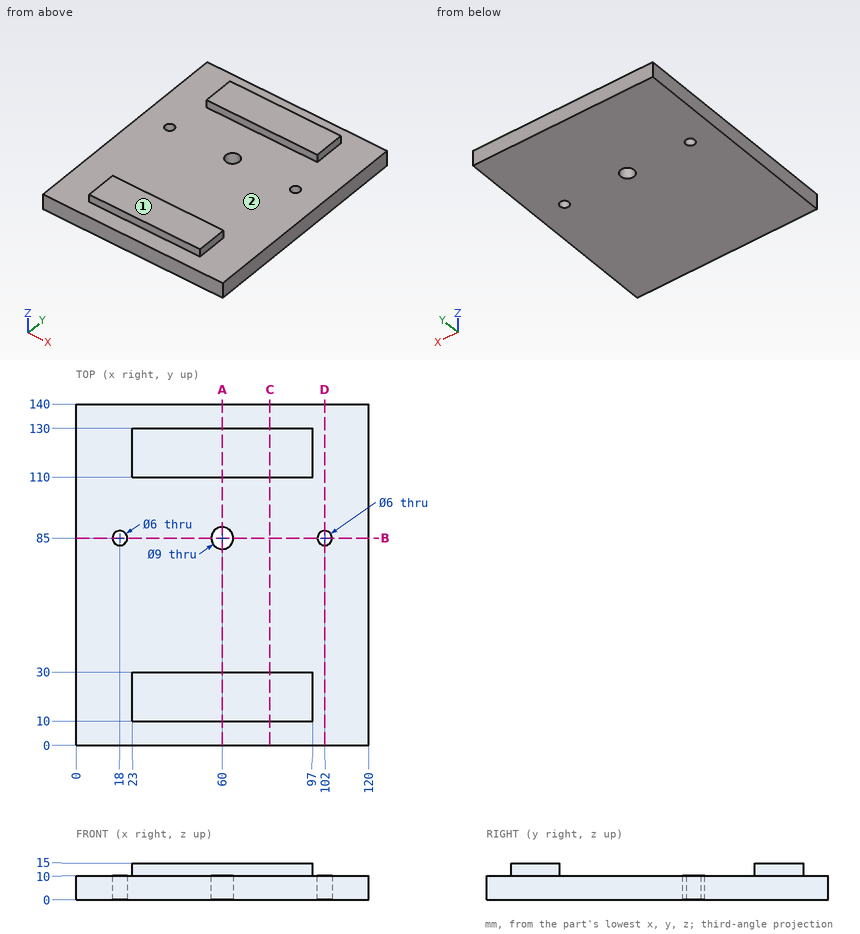
Could you check a few things on this drawing? It's one solid part, dimensions in mm from its lowest x, y, z. Round coordinates to 2 decimals unless told otherwise and drop trailing zeros. Loops run counter-clockwise (first coordinate to the right, second up) from the corner with the lowest first, then second, coordinate; pieces in that order, holes last.
Q1. I want a section at A-A (x = 60). Write out the boundary of the cut face in (y, z), and give its area (3 significant figures).
Q2. I want a section at B-B (y = 85). Write out the boundary of the cut face in (x, z).
Q3. Thinking about a two-plate mould opening in Y: for the marked faces 1 and 2, which applies, pulls with the +Y half, pulls with the -Y half, needs draft (parallel to the pull), parting line crosses it, or undercut?
Q4. For P1, Ø1.5, axis at x = 77, y = 118, coming from the -Z side; P2, Ø1.5, axis at y = 22.5, z = 11.5, coming from the +X side; P3, Ø4, axis at x = 58.5, z = 13.5, coming from the +Y side; P4, Ø2.5, axis at y = 117, z = 12.5, coming from the -X side, each with a flat end and sliding along its axis, tell me the tip position at first contact or that it passes through.
Q5. Please list where these lines run through material, in increasing order: L1, parallel to Y at x = 102, z = 5.25; L2, parallel to Y at x = 43.5, z = 11.25; L3, parallel to X at y = 23, z = 12.5.
Q6. I want a section at D-D (x = 102). Write out the boundary of the cut face in (y, z).
Q7. I want a section at C-C (x = 79.5). Write out the boundary of the cut face in (y, z), and give its area (3 significant figures).
Answer below:
1. outline: (0, 0) - (80.5, 0) - (80.5, 10) - (30, 10) - (30, 15) - (10, 15) - (10, 10) - (0, 10) - close; (89.5, 0) - (140, 0) - (140, 10) - (130, 10) - (130, 15) - (110, 15) - (110, 10) - (89.5, 10) - close
1. area: 1,510 mm2
2. outline: (0, 0) - (15, 0) - (15, 10) - (0, 10) - close; (21, 0) - (55.5, 0) - (55.5, 10) - (21, 10) - close; (64.5, 0) - (99, 0) - (99, 10) - (64.5, 10) - close; (105, 0) - (120, 0) - (120, 10) - (105, 10) - close
3. face 1: needs draft
3. face 2: undercut
4. P1: stops at z = 0
4. P2: stops at x = 97
4. P3: stops at y = 130
4. P4: stops at x = 23
5. L1: y = 0 to 82, 88 to 140
5. L2: y = 10 to 30, 110 to 130
5. L3: x = 23 to 97
6. outline: (0, 0) - (82, 0) - (82, 10) - (0, 10) - close; (88, 0) - (140, 0) - (140, 10) - (88, 10) - close
7. outline: (0, 0) - (140, 0) - (140, 10) - (130, 10) - (130, 15) - (110, 15) - (110, 10) - (30, 10) - (30, 15) - (10, 15) - (10, 10) - (0, 10) - close
7. area: 1,600 mm2
